```python
from build123d import *

# Parameters (mm, degrees)
SKETCH1_R           = 2.25
BOSS_EXTRUDE1_DEPTH = 3.5
SKETCH2_R           = 1.5
BOSS_EXTRUDE2_DEPTH = 26
BOSS_EXTRUDE3_START = 3.5
SKETCH3_R           = 2.25
BOSS_EXTRUDE3_DEPTH = 3.5
CHAMFER1_SIZE       = 1


with BuildPart() as part:
    # Sketch1 → Boss-Extrude1 (new body)
    with BuildSketch(Plane(origin=(0, 0, 0), x_dir=(1, 0, 0), z_dir=(0, 1, 0))):
        with Locations(Location((0, 0, 0), (0, 0, 270))):
            Circle(SKETCH1_R)
    extrude(amount=BOSS_EXTRUDE1_DEPTH)

    # Sketch2 → Boss-Extrude2 (add)
    with BuildSketch(Plane.XZ):
        with Locations(Location((0, 0, 0), (0, 0, 90))):
            Circle(SKETCH2_R)
    extrude(amount=BOSS_EXTRUDE2_DEPTH)

    # Sketch3 → Boss-Extrude3 (add)
    with BuildSketch(Plane.XZ.offset(26).offset(BOSS_EXTRUDE3_START)):
        with Locations(Location((0, 0, 0), (0, 0, 90))):
            Circle(SKETCH3_R)
    extrude(amount=-BOSS_EXTRUDE3_DEPTH)

    # Chamfer1
    chamfer1_edges = [part.edges().sort_by_distance(p)[0] for p in [
        (0, -29.5, -2.25),
        (0, 3.5, -2.25),
    ]]
    chamfer(chamfer1_edges, length=CHAMFER1_SIZE)


solid = part.part
```
Here's how the part is built. I have some questions about the finished solid (model axes, mm). A direction names the side the tool comes from. Coordinates: 2 decimals unless noted, no trailing zeros. Order: outer loops, then holes, each group sorted by start corner. A loop starts at its lowest first (then second) coordinate and runs counter-clockwise, first axis right, second up. Notation, with made-up numbers: (11.5, -4) - (21.5, -4) arc R21 ccw to (21.5, 15) - close; hole circle Ø6 at (78.25, 66). An arc over 180 degrees is marked (long way). One line per question, with ' | ' between items. Start each with the question number.
1. Please list where these lines run through material, in increasing order: line 1 along Y through (x, z) = (1.6, -0.2); line 2 along Y through (x, z) = (-2, -0.95); line 3 along Z through (x, y) = (0.15, -4.5). Write a range as [from, to].
2. If we section it at B-B (x = 0): Write out the boundary of the cut face in (y, z).
3. Which directions (+Z, -Z, +X, -X, +Y, -Y) give clear straight access to the entire face, cutting with the end or side of a thin tool? Please do faces 1 (the cylindrical face through (-0.45, -12.82, 1.43)), 2 (the cylindrical face through (-0.676, -27.268, 2.146)).
4. If we section it at C-C (y = -10.5): Write out the boundary of the cut face in (x, z).
5. If we section it at A-A (z = 0): Write out the boundary of the cut face in (x, y).
6. If we mould it in two halves opening along Y, with no side actions, what happens to faces 3 (the cylindrical face through (0.676, 1.232, 2.146)), 4 (the flat face through (0, 3.5, 0)), 5 (the flat face through (0, 0, -2))? For each: released by +Y, released by -Y, zero draft, split by the parting line, or undercut.
7. I'm going to push flat-ended pins straight in: pin 1 Ø1 at (y, z) = (-23, 1) entering from +X; pin 2 Ø1 at (y, z) = (-12.5, -0.5) entering from -X. Where does each tip first touch, or does it pass through?
Model answer:
1) line 1: y = [-29.14, -26], [0, 3.14] | line 2: y = [-28.54, -26], [0, 2.54] | line 3: z = [-1.49, 1.49]
2) outline: (-29.5, -1.25) - (-28.5, -2.25) - (-26, -2.25) - (-26, -1.5) - (0, -1.5) - (0, -2.25) - (2.5, -2.25) - (3.5, -1.25) - (3.5, 1.25) - (2.5, 2.25) - (0, 2.25) - (0, 1.5) - (-26, 1.5) - (-26, 2.25) - (-28.5, 2.25) - (-29.5, 1.25) - close
3) face 1: none | face 2: +Y, -Y
4) outline: circle Ø3 at (0, 0)
5) outline: (-2.25, -28.5) - (-1.25, -29.5) - (1.25, -29.5) - (2.25, -28.5) - (2.25, -26) - (1.5, -26) - (1.5, 0) - (2.25, 0) - (2.25, 2.5) - (1.25, 3.5) - (-1.25, 3.5) - (-2.25, 2.5) - (-2.25, 0) - (-1.5, 0) - (-1.5, -26) - (-2.25, -26) - close
6) face 3: zero draft | face 4: released by +Y | face 5: undercut
7) pin 1: stops at x = 1.41 | pin 2: stops at x = -1.5
